Geometry: final body of the model. Coordinates: model frame, mm. Coordinates: 2 decimals unless noted, no trailing zeros. Write each loop counter-clockwise with the first axis right and the second up, starting at its lowest first coordinate (ties: lowest second). Pieces come first, ordered by that corner, then holes. Notation, with made-up numbers: (56.5, 48.5) -> (97.5, 48.5) arc R27 cw to (97.5, 74.5) -> close; hole circle Ø11 at (3, 43.5). An arc over 180 degrees is marked (long way). Answer as a JSON object with one key per item and string values. Group by question number.
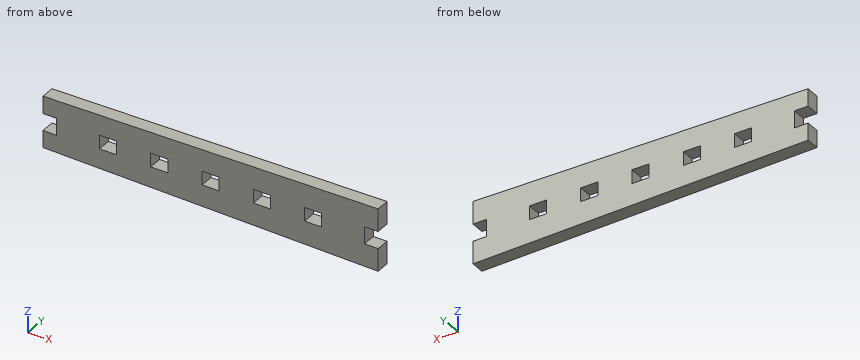
```python
from build123d import *

# Parameters (mm, degrees)
BOSS_EXTRUDE1_DEPTH = 5.08
SKETCH2_W           = 6.35
SKETCH2_H           = 5.08
CUT_EXTRUDE1_DEPTH  = 6.08
LPATTERN1_COUNT     = 5
LPATTERN1_PITCH     = 19.05


with BuildPart() as part:
    # Sketch1 → Boss-Extrude1 (new body)
    with BuildSketch(Plane(origin=(0, 0, 0), x_dir=(1, 0, 0), z_dir=(0, 1, 0))):
        Polygon((-0.444494962, 12.618026496), (-0.444494962, 18.96894547), (124.014769965, 21.086442969), (124.014769965, 12.704442969), (118.934769965, 12.704442969), (118.934769965, 6.354442969), (124.014769965, 6.354442969), (124.014769965, -2.027557031), (-0.445230035, -0.081054515), (-0.445230035, 6.354442969), (4.634769965, 6.354442969), (4.634769965, 12.704442969), align=None)
    extrude(amount=BOSS_EXTRUDE1_DEPTH)

    # Sketch2 → Cut-Extrude1 (cut, through all)
    with BuildSketch(Plane(origin=(0, 5.08, 0), x_dir=(1, 0, 0), z_dir=(0, 1, 0))):
        with Locations((23.684769965, 9.529442969)):
            Rectangle(SKETCH2_W, SKETCH2_H)
    cut_extrude1 = extrude(amount=-CUT_EXTRUDE1_DEPTH, mode=Mode.SUBTRACT)

    # LPattern1: Cut-Extrude1 ×5
    with Locations(*[(i * LPATTERN1_PITCH, 0, 0) for i in range(1, LPATTERN1_COUNT)]):
        add(cut_extrude1, mode=Mode.SUBTRACT)


solid = part.part
```
Item 1: Ray query, L1, parallel to X at y = 2.2, z = -11.75; L2, parallel to Z at x = 78, y = 4.45; L3, parallel to X at y = 3.9, z = -12.5. Return the intervals inside material, ascending. Write a range as [from, to].
Item 2: Section C-C on z = -9. Output: boundary loops of the cut face in (x, y).
Item 3: Section A-A on y = 3.2. Give the number of separate pieces and of enclosed holes in the cut face, then the cut area to 3 significant figures.
Item 4: Contact query for flat-ended pins moving along their axis: pin 1 (2.5 mm diameter, centred on x = 42.5, y = 3.5, fed in from -Z); pin 2 (1.5 mm diameter, centred on x = 82, y = 3, fed in from -Z); pin 3 (2.5 mm diameter, centred on y = 3, z = -10, fed in from -X). Output: stop coordinate, or through.
Item 5: Section D-D on x = 42. Output: boundary loops of the cut face in (y, z).
Item 6: Section B-B on x = 98. Output: boundary loops of the cut face in (y, z), then the cut area to 3 significant figures.
Answer sheet:
{
 "1": {"L1": "x = [4.63, 20.51], [26.86, 39.56], [45.91, 58.61], [64.96, 77.66], [84.01, 96.71], [103.06, 118.93]", "L2": "z = [-20.3, -12.07], [-6.99, 1.31]", "L3": "x = [4.63, 118.93]"},
 "2": {"outline": "(4.63, 0) -> (20.51, 0) -> (20.51, 5.08) -> (4.63, 5.08) -> close; (26.86, 0) -> (39.56, 0) -> (39.56, 5.08) -> (26.86, 5.08) -> close; (45.91, 0) -> (58.61, 0) -> (58.61, 5.08) -> (45.91, 5.08) -> close; (64.96, 0) -> (77.66, 0) -> (77.66, 5.08) -> (64.96, 5.08) -> close; (84.01, 0) -> (96.71, 0) -> (96.71, 5.08) -> (84.01, 5.08) -> close; (103.06, 0) -> (118.93, 0) -> (118.93, 5.08) -> (103.06, 5.08) -> close"},
 "3": {"separate pieces": "1", "enclosed holes": "5", "area": "2,400 mm^2"},
 "4": {"pin 1": "stops at z = -19.72", "pin 2": "stops at z = -20.38", "pin 3": "stops at x = 4.63"},
 "5": {"outline": "(0, -19.69) -> (5.08, -19.69) -> (5.08, -12.07) -> (0, -12.07) -> close; (0, -6.99) -> (5.08, -6.99) -> (5.08, 0.74) -> (0, 0.74) -> close"},
 "6": {"outline": "(0, -20.64) -> (5.08, -20.64) -> (5.08, -12.07) -> (0, -12.07) -> close; (0, -6.99) -> (5.08, -6.99) -> (5.08, 1.62) -> (0, 1.62) -> close", "area": "87.3 mm^2"}
}
